Input: part model. Units: mm. Frame: model coordinates. Face numbers are marked on the shaded views. Give positions to 0.01 mm unless a question says otherwise; leave off trailing zeros. Loops run counter-clockwise (first coordinate to the right, second up) from the corner with the lowest first, then second, coordinate; pieces in that order, holes last. Notation, with made-up numbers: (45.5, -1.75) - (50.5, -1.75) arc R15 ccw to (50.5, 5.25) - close; hole circle Ø5 at (55, -33.5). An arc over 180 degrees is marked (long way). One line per item, written item: value.
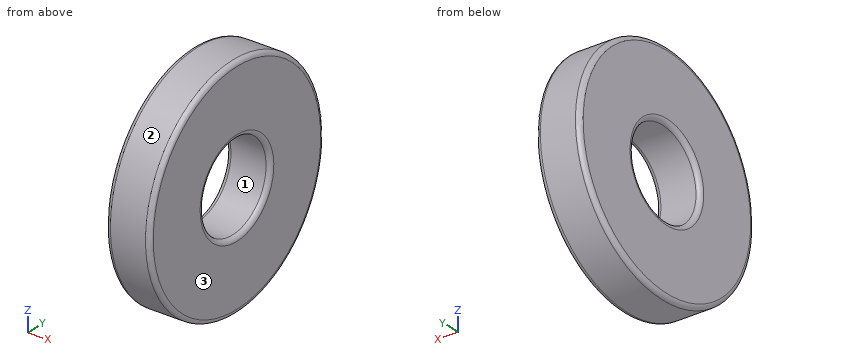
from build123d import *


with BuildPart() as f1:
    # F0 (on Front) → F1 (revolve)
    with BuildSketch(Plane.XZ):
        with BuildLine():
            Line((5.08, 33.02), (-5.08, 33.02))
            ThreePointArc((-5.08, 33.02), (-5.978026, 32.648026), (-6.35, 31.75))
            Line((-6.35, 31.75), (-6.35, 13.97))
            ThreePointArc((-6.35, 13.97), (-5.978026, 13.071974), (-5.08, 12.7))
            Line((-5.08, 12.7), (5.08, 12.7))
            ThreePointArc((5.08, 12.7), (5.978026, 13.071974), (6.35, 13.97))
            Line((6.35, 13.97), (6.35, 31.75))
            ThreePointArc((6.35, 31.75), (5.978026, 32.648026), (5.08, 33.02))
        make_face()
    revolve(axis=Axis((-17.721478, 0, 0), (-1, 0, 0)))


solid = f1.part
Item 1: Pin query (flat end, axial travel): P1, Ø1.5, axis at x = 0.5, z = 10.5, coming from the +Y side; P2, Ø1.5, axis at x = -3, y = -23, coming from the +Z side; P3, Ø2, axis at x = -4, z = -10, coming from the -Y side. Return the tip coordinate at first contact, or that it passes through.
Verdict:
P1: stops at y = 31.55
P2: stops at z = 24.4
P3: stops at y = -31.77
Item 2: Material intervals for L1, parallel to Y at x = 2.25, z = 0; L2, parallel to Z at x = -3.25, y = 1; L3, parallel to Y at x = 2.5, z = 3.5, sorted ascending.
Verdict:
L1: y = -33.02 to -12.7, 12.7 to 33.02
L2: z = -33 to -12.66, 12.66 to 33
L3: y = -32.83 to -12.21, 12.21 to 32.83
Item 3: Section C-C, the plane x = 0. Output: boundary loops of the cut face in (y, z).
Verdict:
outline: circle Ø66.04 at (0, 0); hole circle Ø25.4 at (0, 0)
Item 4: Draft query along Z for the marked faces 1, 2 and 3. Return one class per face: pulls with the +Z half, pulls with the -Z half, needs draft (parallel to the pull), parting line crosses it, or undercut.
Verdict:
face 1: undercut
face 2: parting line crosses it
face 3: needs draft
Item 5: Section A-A, the plane y = 0. Output: boundary loops of the cut face in (x, z).
Verdict:
outline: (-6.35, -31.75) arc R1.27 ccw to (-5.08, -33.02) - (5.08, -33.02) arc R1.27 ccw to (6.35, -31.75) - (6.35, -13.97) arc R1.27 ccw to (5.08, -12.7) - (-5.08, -12.7) arc R1.27 ccw to (-6.35, -13.97) - close; (-6.35, 13.97) arc R1.27 ccw to (-5.08, 12.7) - (5.08, 12.7) arc R1.27 ccw to (6.35, 13.97) - (6.35, 31.75) arc R1.27 ccw to (5.08, 33.02) - (-5.08, 33.02) arc R1.27 ccw to (-6.35, 31.75) - close
